Part print with two shaded views. Sizes in mm from the minimum x, y, z corner. A direction names the side the tool comes from. Give positions to 0.01 mm unless a question says otherwise; leave off trailing zeros. Order: outer loops, then holes, each group sorted by start corner. A loop starts at its lowest first (then second) coordinate and runs counter-clockwise, first axis right, second up. Notation, with made-up numbers: M 0,27.5 L 59,27.5 A22 cw 59,57.5 Z; hole C -20.5,0.25 d6. An arc over 180 degrees is marked long. Return JSON: item names as keys, results as strings. Group by question number.
1. Slice it at B-B on y = 14. List the corners of the cut face in (x, z).
2. Slice it at D-D on x = 11.25. List the corners of the cut face in (y, z), then the cut area to 3 significant figures.
3. Wall check: probe 1 along X at (y, z) = (10, 12.55); probe 2 along Y at (x, z) = (7.5, 12.8); probe 3 along Z at (x, y) = (3, 9.75). Give the ranges that are in metal, low to high. Write a range as [from, to].
4. Two-plate mould, pull along Y, no slides. Class the marked faces 1, 2 and 3: released by +Y, released by -Y, zero draft, split by the parting line, or undercut.
5. 3-axis set-ups, long thin cutter, end or side, ignore diameter. For the marked faces 4 and 5: which of +Z, -Z, +X, -X, +Y, -Y reach the whole face in a straight line?
6. Slice it at A-A on x = 7.5. List the corners of the cut face in (y, z).
7. Slice it at C-C on z = 11. List the corners of the cut face in (x, y).
8. Pin check, flat tips, straight feed: pin 1 (3 mm diameter, centred on x = 4, z = 4, fed in from +Y); pin 2 (1 mm diameter, centred on x = 4.5, y = 6.5, fed in from +Z); pin 3 (1.5 mm diameter, centred on x = 3, y = 14, fed in from -Z); pin 4 (5 mm diameter, centred on y = 13.5, z = 11.5, fed in from +X). Stop position of each tip, or through.
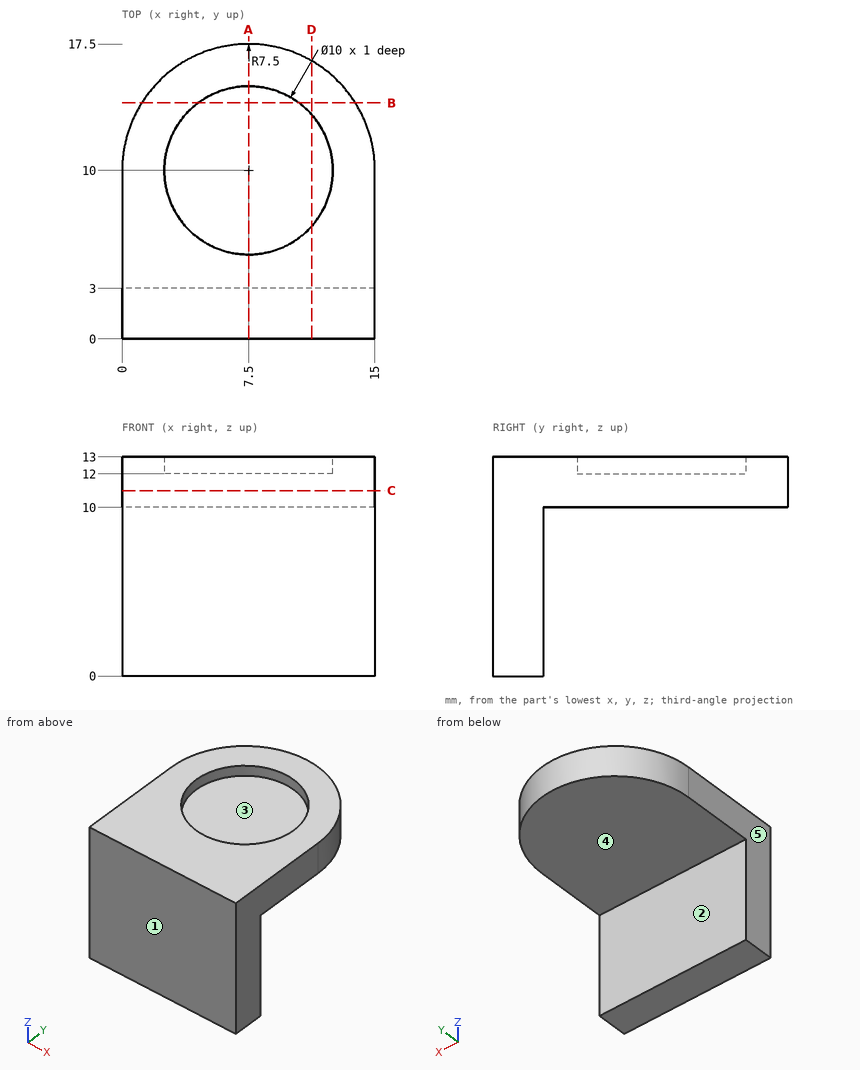
Result:
{
 "1": {"outline": "M 1.16,10 L 13.84,10 L 13.84,13 L 10.5,13 L 10.5,12 L 4.5,12 L 4.5,13 L 1.16,13 Z"},
 "2": {"outline": "M 0,0 L 3,0 L 3,10 L 16.5,10 L 16.5,13 L 13.31,13 L 13.31,12 L 6.69,12 L 6.69,13 L 0,13 Z", "area": "72.9 mm2"},
 "3": {"probe 1": "x = [0, 2.5], [12.5, 15]", "probe 2": "y = [0, 5], [15, 17.5]", "probe 3": "z = [10, 12]"},
 "4": {"face 1": "released by -Y", "face 2": "released by +Y", "face 3": "undercut"},
 "5": {"face 4": "-Z, +X, -X, +Y", "face 5": "+Z, -Z, -X, +Y, -Y"},
 "6": {"outline": "M 0,0 L 3,0 L 3,10 L 17.5,10 L 17.5,13 L 15,13 L 15,12 L 5,12 L 5,13 L 0,13 Z"},
 "7": {"outline": "M 0,0 L 15,0 L 15,10 A7.5 ccw 0,10 Z"},
 "8": {"pin 1": "stops at y = 3", "pin 2": "stops at z = 13", "pin 3": "stops at z = 10", "pin 4": "stops at x = 14.93"}
}
